```python
from build123d import *

# Parameters (mm, degrees)
EXTRUDE_THIN1_DEPTH = 10
EXTRUDE_THIN2_DEPTH = 10


# Read off the part's stored shape, not the designer's step: Extrude-Thin1
with BuildPart() as part:
    # Extrude-Thin1 outline → Extrude-Thin1 (new body)
    with BuildSketch(Plane.XY):
        Polygon((-9.314102564, -0.45), (-9.314102564, -12.75), (9.185897436, -12.75), (9.185897436, -4), (7.685897436, -4), (7.685897436, -11.25), (-7.814102564, -11.25), (-7.814102564, -0.75), (4.685897436, -0.75), (4.685897436, -10), (6.185897436, -10), (6.185897436, 0.75), (-9.014102564, 0.75), align=None)
    extrude(amount=EXTRUDE_THIN1_DEPTH)

    # Sketch2 → Extrude-Thin2 (add)
    with BuildSketch(Plane.XY.offset(10)):
        with BuildLine():
            Line((-9.014102564, 0.75), (-9.314102564, -0.45))
            Line((-9.314102564, -0.45), (-9.314102564, -7.5))
            ThreePointArc((-9.314102564, -7.5), (-9.592351122, -8.171751442), (-10.264102564, -8.45))
            Line((-10.264102564, -8.45), (-10.314102564, -8.45))
            Line((-10.314102564, -8.45), (-10.314102564, -7.95))
            Line((-10.314102564, -7.95), (-10.264102564, -7.95))
            ThreePointArc((-10.264102564, -7.95), (-9.945904513, -7.818198052), (-9.814102564, -7.5))
            Line((-9.814102564, -7.5), (-9.814102564, -0.388447187))
            Line((-9.814102564, -0.388447187), (-9.499173814, 0.871267813))
            Line((-9.499173814, 0.871267813), (-9.014102564, 0.75))
        make_face()
    extrude(amount=-EXTRUDE_THIN2_DEPTH)


solid = part.part
```
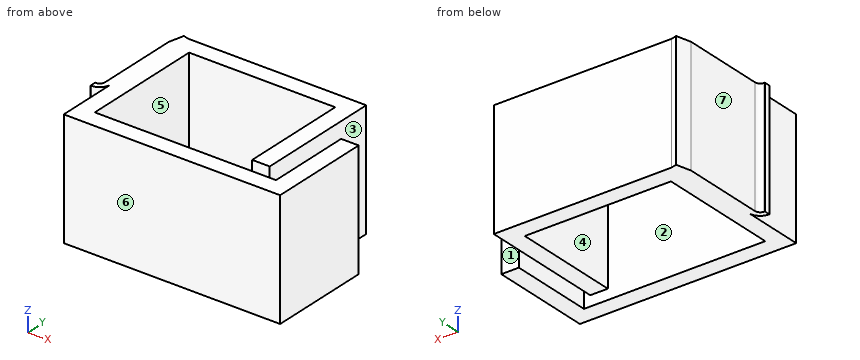
Verification items for the finished model (mm, model axes). Face numbers are marked on the shaded views. A direction names the side the tool comes from. Round coordinates to 2 decimals unless told otherwise and drop trailing zeros. Order: outer loops, then holes, each group sorted by start corner. A loop starts at its lowest first (then second) coordinate and runs counter-clockwise, first axis right, second up. Notation, with made-up numbers: (84, -23.75) - (101, -23.75) arc R27 ccw to (101, -5.75) - close; hole circle Ø9 at (47.5, 81). An arc over 180 degrees is marked (long way). Use CSV: the item, a comma, the result in double quotes.
(1) Section check A-A on y = -6.5. Record the boundary of the cut face in (x, z).
Entries:
outline,"(-9.81, 0) - (-7.81, 0) - (-7.81, 10) - (-9.81, 10) - close; (4.69, 0) - (6.19, 0) - (6.19, 10) - (4.69, 10) - close; (7.69, 0) - (9.19, 0) - (9.19, 10) - (7.69, 10) - close"
(2) Section check D-D on y = -3.75. Record the boundary of the cut face in (x, z).
Entries:
outline,"(-9.81, 0) - (-7.81, 0) - (-7.81, 10) - (-9.81, 10) - close; (4.69, 0) - (6.19, 0) - (6.19, 10) - (4.69, 10) - close"
(3) Gauge pin test, flat ends, axial feed: pin 1 Ø1.5 at (x, z) = (-2, 4.5) entering from +Y; pin 2 Ø5.5 at (y, z) = (-4.5, 6) entering from -X; pin 3 Ø2.5 at (y, z) = (-10.5, 2.5) entering from -X. Record the tip position at first contact, or that the pin passes through.
Entries:
pin 1,"y = 0.75"
pin 2,"x = -9.81"
pin 3,"x = -9.31"
(4) Section check B-B on x = -2.5. Record the boundary of the cut face in (y, z).
Entries:
outline,"(-12.75, 0) - (-11.25, 0) - (-11.25, 10) - (-12.75, 10) - close; (-0.75, 0) - (0.75, 0) - (0.75, 10) - (-0.75, 10) - close"
(5) Mould release check, pull along X, two halves, no side actions. Record for the marked faces 4, 5, 6 and 7: released by +X, released by -X, zero draft, split by the parting line, or undercut.
Entries:
face 4,"undercut"
face 5,"undercut"
face 6,"zero draft"
face 7,"released by -X"
(6) Access from +Z, -Z, +X, -X, +Y, -Y to the whole of each face (thin tool, end or side, straight path). Record for the marked faces 1, 2 and 3.
Entries:
face 1,"+Z, -Z, +X, +Y"
face 2,"+Z, -Z"
face 3,"+Z, -Z, +Y"
(7) Section check C-C on z = 8.5. Record the boundary of the cut face in (x, y).
Entries:
outline,"(-10.31, -8.45) - (-10.26, -8.45) arc R0.95 ccw to (-9.31, -7.5) - (-9.31, -12.75) - (9.19, -12.75) - (9.19, -4) - (7.69, -4) - (7.69, -11.25) - (-7.81, -11.25) - (-7.81, -0.75) - (4.69, -0.75) - (4.69, -10) - (6.19, -10) - (6.19, 0.75) - (-9.01, 0.75) - (-9.5, 0.87) - (-9.81, -0.39) - (-9.81, -7.5) arc R0.45 cw to (-10.26, -7.95) - (-10.31, -7.95) - close"
(8) Thickness scan on probe 1 along X at (y, z) = (-6, 7.25); probe 2 along Y at (x, z) = (-5.25, 6.5); probe 3 along X at (y, z) = (-3.5, 5.25). Record the ranges inside material, lowest first. Write a range as from..to.
Entries:
probe 1,"-9.81..-7.81, 4.69..6.19, 7.69..9.19"
probe 2,"-12.75..-11.25, -0.75..0.75"
probe 3,"-9.81..-7.81, 4.69..6.19"
